from build123d import *

# Parameters (mm, degrees)
SKETCH1_W           = 72
SKETCH1_H           = 75
SKETCH1_R           = 2.75
SKETCH1_R_2         = 6.25
BOSS_EXTRUDE3_DEPTH = 9
FILLET1_R           = 4
SKETCH4_R           = 16.25
CUT_EXTRUDE2_DEPTH  = 4
SKETCH3_R           = 6.25
CUT_EXTRUDE3_DEPTH  = 3.5


with BuildPart() as part:
    # Sketch1 → Boss-Extrude3 (new body)
    with BuildSketch(Plane(origin=(0, 0, 0), x_dir=(1, 0, 0), z_dir=(0, 1, 0))):
        with Locations((30.01, -31)):
            Rectangle(SKETCH1_W, SKETCH1_H)
        Circle(SKETCH1_R, mode=Mode.SUBTRACT)
        with Locations((60.02, 0)):
            Circle(SKETCH1_R, mode=Mode.SUBTRACT)
        with Locations((60.02, -62)):
            Circle(SKETCH1_R, mode=Mode.SUBTRACT)
        with Locations((0, -62)):
            Circle(SKETCH1_R, mode=Mode.SUBTRACT)
        with Locations((30.01, -31)):
            Circle(SKETCH1_R_2, mode=Mode.SUBTRACT)
        with Locations((14.100097423, -15.090097423)):
            Circle(SKETCH1_R, mode=Mode.SUBTRACT)
        with Locations((14.100097423, -46.909902577)):
            Circle(SKETCH1_R, mode=Mode.SUBTRACT)
        with Locations((45.919902577, -46.909902577)):
            Circle(SKETCH1_R, mode=Mode.SUBTRACT)
        with Locations((45.919902577, -15.090097423)):
            Circle(SKETCH1_R, mode=Mode.SUBTRACT)
    extrude(amount=BOSS_EXTRUDE3_DEPTH)

    # Fillet1
    fillet1_edges = [part.edges().sort_by_distance(p)[0] for p in [
        (66.01, 4.5, 68.5),
        (-5.99, 4.5, 68.5),
        (-5.99, 4.5, -6.5),
        (66.01, 4.5, -6.5),
    ]]
    fillet(fillet1_edges, radius=FILLET1_R)

    # Sketch4 → Cut-Extrude2 (cut)
    with BuildSketch(Plane.XZ):
        with Locations((30.01, 31)):
            Circle(SKETCH4_R)
    extrude(amount=-CUT_EXTRUDE2_DEPTH, mode=Mode.SUBTRACT)

    # Sketch3 → Cut-Extrude3 (cut)
    with BuildSketch(Plane(origin=(0, 9, 0), x_dir=(1, 0, 0), z_dir=(0, 1, 0))):
        with Locations((14.100097423, -46.909902577)):
            Circle(SKETCH3_R)
        with Locations((14.100097423, -15.090097423)):
            Circle(SKETCH3_R)
        with Locations((45.919902577, -15.090097423)):
            Circle(SKETCH3_R)
        with Locations((45.919902577, -46.909902577)):
            Circle(SKETCH3_R)
    extrude(amount=-CUT_EXTRUDE3_DEPTH, mode=Mode.SUBTRACT)


solid = part.part
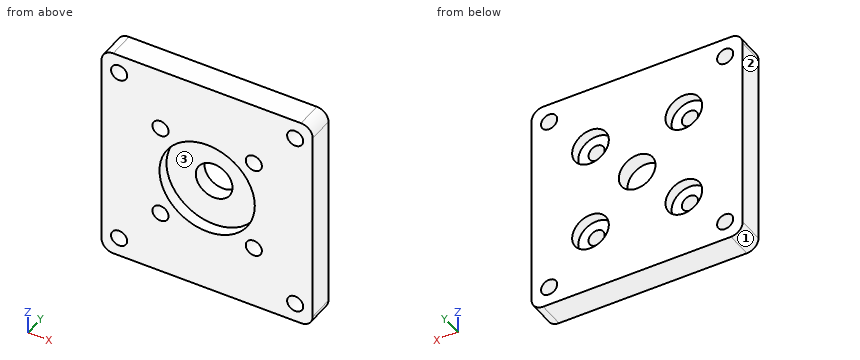
For this review, take the finished solid that the model builds, in its own axes (mm). Face numbers are marked on the shaded views. Coordinates: 2 decimals unless noted, no trailing zeros. Loops run counter-clockwise (first coordinate to the right, second up) from the corner with the lowest first, then second, coordinate; pieces in that order, holes last. Notation, with made-up numbers: (33.25, -13) - (73.25, -13) arc R30 cw to (73.25, 16) - close; hole circle Ø5 at (23.5, 76). An arc over 180 degrees is marked (long way). Return JSON: item names as keys, results as strings.
Item 1: Take a section at D-D (z = 31). Give the boundary of the cut face in (x, y), then the cut area to 4 significant figures.
Determined:
{"outline": "(-5.99, 0) - (13.76, 0) - (13.76, 4) - (23.76, 4) - (23.76, 9) - (-5.99, 9) - close; (36.26, 4) - (46.26, 4) - (46.26, 0) - (66.01, 0) - (66.01, 9) - (36.26, 9) - close", "area": "455.5 mm2"}
Item 2: Take a section at C-C (x = 0). Give the boundary of the cut face in (y, z), then the cut area to 3 significant figures.
Determined:
{"outline": "(0, -6.5) - (9, -6.5) - (9, -2.75) - (0, -2.75) - close; (0, 2.75) - (9, 2.75) - (9, 59.25) - (0, 59.25) - close; (0, 64.75) - (9, 64.75) - (9, 68.5) - (0, 68.5) - close", "area": "576 mm2"}
Item 3: Mouldability with a two-part tool opening along Z and no side actions: class the marked faces 1, 2 and 3 as pulls with the +Z half, pulls with the -Z half, needs draft (parallel to the pull), parting line crosses it, or undercut.
Determined:
{"face 1": "pulls with the -Z half", "face 2": "needs draft", "face 3": "undercut"}
Item 4: Insertion check: pin 1 (7.5 mm diameter, centred on x = 14.1, z = 15.09, fed in from +Y); pin 2 (8 mm diameter, centred on x = 53, z = 17.5, fed in from -Y); pin 3 (14.5 mm diameter, centred on x = 30.01, z = 31, fed in from -Y). Each pin has a flat end and moves straight along its axis. Give the tip position at first contact, or say it passes through.
Determined:
{"pin 1": "stops at y = 5.5", "pin 2": "stops at y = 0", "pin 3": "stops at y = 4"}
Item 5: Take a section at B-B (z = 62). Give the boundary of the cut face in (x, y).
Determined:
{"outline": "(-5.99, 0) - (-2.75, 0) - (-2.75, 9) - (-5.99, 9) - close; (2.75, 0) - (57.27, 0) - (57.27, 9) - (2.75, 9) - close; (62.77, 0) - (66.01, 0) - (66.01, 9) - (62.77, 9) - close"}
Item 6: For line 1 (X direction, y = 2.25, z = 62); line 2 (X direction, y = 5, z = -1); line 3 (Z direction, x = 16, y = 0.75), list the stretches that pass through material, from the lowest coordinate up.
Determined:
{"line 1": "x = -5.99 to -2.75, 2.75 to 57.27, 62.77 to 66.01", "line 2": "x = -5.99 to -2.56, 2.56 to 57.46, 62.58 to 66.01", "line 3": "z = -6.5 to 13.1, 17.08 to 22.77, 39.23 to 44.92, 48.9 to 68.5"}
Item 7: Take a section at A-A (x = 30.01). Give the boundary of the cut face in (y, z).
Determined:
{"outline": "(0, -6.5) - (9, -6.5) - (9, 24.75) - (4, 24.75) - (4, 14.75) - (0, 14.75) - close; (0, 47.25) - (4, 47.25) - (4, 37.25) - (9, 37.25) - (9, 68.5) - (0, 68.5) - close"}
